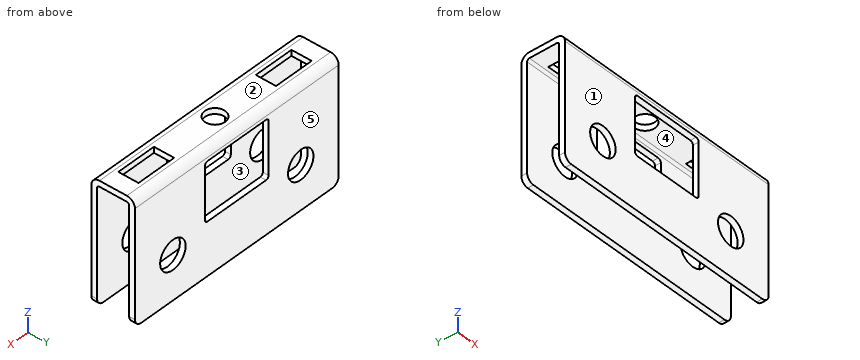
```python
from build123d import *

# Parameters (mm, degrees)
SKETCH1_W                      = 80
SKETCH1_H                      = 2
BASE_FLANGE1_DEPTH             = 5.55
EDGE_FLANGE1_STRIP_W           = 9.6
EDGE_FLANGE1_STRIP_H           = 2
EDGE_FLANGE1_STRIP_CUT_DEPTH   = 80
EDGE_FLANGE1_STRIP_2_W         = 9.6
EDGE_FLANGE1_STRIP_2_H         = 2
EDGE_FLANGE1_STRIP_CUT_2_DEPTH = 80
EDGE_FLANGE1_DEPTH             = 80
EDGE_FLANGE1_BEND_DEPTH        = 80
SKETCH12_R                     = 3.5
SKETCH12_W                     = 14
SKETCH12_H                     = 7
CUT_EXTRUDE1_DEPTH             = 59.561185951
SKETCH13_W                     = 25
SKETCH13_H                     = 20
CUT_EXTRUDE2_DEPTH             = 59.617574157
FILLET1_R                      = 1
FILLET2_R                      = 2.5
SKETCH15_R                     = 5
CUT_EXTRUDE3_DEPTH             = 59.617574157


# Sheet-metal steps are written as plain solids
with BuildPart() as part:
    # Sketch1 → Base-Flange1 (new, symmetric)
    with BuildSketch(Plane(origin=(0, 0, 0), x_dir=(1, 0, 0), z_dir=(0, 1, 0))):
        with Locations((0, -1)):
            Rectangle(SKETCH1_W, SKETCH1_H)
    extrude(amount=BASE_FLANGE1_DEPTH, both=True)

    # Edge-Flange1 strip (across the edge) → Edge-Flange1 strip cut (cut)
    with BuildSketch(Plane(origin=(40, -5.55, 0), x_dir=(0, 1, 0), z_dir=(-1, 0, 0))):
        with Locations((-4, -1)):
            Rectangle(EDGE_FLANGE1_STRIP_W, EDGE_FLANGE1_STRIP_H)
    extrude(amount=EDGE_FLANGE1_STRIP_CUT_DEPTH, mode=Mode.SUBTRACT)

    # Edge-Flange1 strip 2 (across the edge) → Edge-Flange1 strip cut 2 (cut)
    with BuildSketch(Plane(origin=(-40, 5.55, 0), x_dir=(0, -1, 0), z_dir=(1, 0, 0))):
        with Locations((-4, -1)):
            Rectangle(EDGE_FLANGE1_STRIP_2_W, EDGE_FLANGE1_STRIP_2_H)
    extrude(amount=EDGE_FLANGE1_STRIP_CUT_2_DEPTH, mode=Mode.SUBTRACT)

    # Edge-Flange1 section (across the edge) → Edge-Flange1 (add)
    with BuildSketch(Plane(origin=(40, -5.55, 0), x_dir=(0, 1, 0), z_dir=(-1, 0, 0))):
        with BuildLine():
            Line((-2, 0.8), (-2, 40.1))
            Line((-2, 40.1), (0, 40.1))
            Line((0, 40.1), (0, 0.8))
            ThreePointArc((0, 0.8), (0.234314575, 0.234314575), (0.8, 0))
            Line((0.8, 0), (0.8, -2))
            ThreePointArc((0.8, -2), (-1.179898987, -1.179898987), (-2, 0.8))
        make_face()
    extrude(amount=EDGE_FLANGE1_DEPTH)

    # Edge-Flange1 section 2 (across the edge) → Edge-Flange1 bend (add)
    with BuildSketch(Plane(origin=(-40, 5.55, 0), x_dir=(0, -1, 0), z_dir=(1, 0, 0))):
        with BuildLine():
            Line((-2, 0.8), (-2, 40.1))
            Line((-2, 40.1), (0, 40.1))
            Line((0, 40.1), (0, 0.8))
            ThreePointArc((0, 0.8), (0.234314575, 0.234314575), (0.8, 0))
            Line((0.8, 0), (0.8, -2))
            ThreePointArc((0.8, -2), (-1.179898987, -1.179898987), (-2, 0.8))
        make_face()
    extrude(amount=EDGE_FLANGE1_BEND_DEPTH)

    # Sketch12 → Cut-Extrude1 (cut, through all)
    with BuildSketch(Plane.XY.offset(2)):
        Circle(SKETCH12_R)
        with Locations((-27, 0)):
            Rectangle(SKETCH12_W, SKETCH12_H)
        with Locations((27, 0)):
            Rectangle(SKETCH12_W, SKETCH12_H)
    extrude(amount=-CUT_EXTRUDE1_DEPTH, mode=Mode.SUBTRACT)

    # Sketch13 → Cut-Extrude2 (cut, through all)
    with BuildSketch(Plane(origin=(0, 7.55, 0), x_dir=(1, 0, 0), z_dir=(0, 1, 0))):
        with Locations((0, 12)):
            Rectangle(SKETCH13_W, SKETCH13_H)
    extrude(amount=-CUT_EXTRUDE2_DEPTH, mode=Mode.SUBTRACT)

    # Fillet1
    fillet1_edges = [part.edges().sort_by_distance(p)[0] for p in [
        (-12.5, -6.55, -2),
        (-12.5, -6.55, -22),
        (12.5, -6.55, -22),
        (12.5, -6.55, -2),
        (-12.5, 6.55, -2),
        (-12.5, 6.55, -22),
        (12.5, 6.55, -22),
        (12.5, 6.55, -2),
    ]]
    fillet(fillet1_edges, radius=FILLET1_R)

    # Fillet2
    fillet2_edges = [part.edges().sort_by_distance(p)[0] for p in [
        (40, -6.55, -40.1),
        (-40, -6.55, -40.1),
        (-40, 6.55, -40.1),
        (40, 6.55, -40.1),
    ]]
    fillet(fillet2_edges, radius=FILLET2_R)

    # Sketch15 → Cut-Extrude3 (cut, through all)
    with BuildSketch(Plane.XZ.offset(7.55)):
        with Locations(Location((25.1, -25, 0), (0, 0, 270))):
            Circle(SKETCH15_R)
        with Locations(Location((-25.1, -25, 0), (0, 0, 270))):
            Circle(SKETCH15_R)
    extrude(amount=-CUT_EXTRUDE3_DEPTH, mode=Mode.SUBTRACT)


solid = part.part
```
Input: part model. Units: mm. Frame: model coordinates. Face numbers are marked on the shaded views. A direction names the side the tool comes from. Give positions to 0.01 mm unless a question says otherwise; leave off trailing zeros. Loops run counter-clockwise (first coordinate to the right, second up) from the corner with the lowest first, then second, coordinate; pieces in that order, holes last.
1) Section query A-A on z = -33. Return the cut outline in (x, y), and give its area (3 significant figures).
A:
outline: (-40, -7.55) - (40, -7.55) - (40, -5.55) - (-40, -5.55) - close; (-40, 5.55) - (40, 5.55) - (40, 7.55) - (-40, 7.55) - close
area: 320 mm2
2) Reachability of the marked faces 4 and 5 from +Z, -Z, +X, -X, +Y, -Y: full face, straight path, thin tool, end or side. Return the list, or none.
A:
face 4: -Z, +X, -X
face 5: +Z, -Z, +X, -X, +Y
3) Mould query, pull axis Y, two halves, no side actions, for the marked faces 1, 2 and 3. Classes: released by +Y, released by -Y, zero draft, split by the parting line, or undercut.
A:
face 1: released by -Y
face 2: zero draft
face 3: undercut
4) Section query B-B on x = -25.1. Return the cut outline in (y, z), and give its area (3 significant figures).
A:
outline: (-7.55, -40.1) - (-5.55, -40.1) - (-5.55, -30) - (-7.55, -30) - close; (-7.55, -20) - (-5.55, -20) - (-5.55, -0.8) arc R0.8 cw to (-4.75, 0) - (-3.5, 0) - (-3.5, 2) - (-4.75, 2) arc R2.8 ccw to (-7.55, -0.8) - close; (3.5, 0) - (4.75, 0) arc R0.8 cw to (5.55, -0.8) - (5.55, -20) - (7.55, -20) - (7.55, -0.8) arc R2.8 ccw to (4.75, 2) - (3.5, 2) - close; (5.55, -40.1) - (7.55, -40.1) - (7.55, -30) - (5.55, -30) - close
area: 134 mm2
5) Contact query for flat-ended pins moving along their axis: pin 1 (12 mm diameter, centred on x = 4, z = -18.5, fed in from +Y); pin 2 (2 mm diameter, centred on x = 24.5, z = 0.5, fed in from -Y); pin 3 (7.5 mm diameter, centred on x = 19, y = -0.5, fed in from -Z); pin 4 (0.6 mm diameter, centred on x = -24, z = 1, fed in from -Y). Output: stop coordinate, or through.
A:
pin 1: stops at y = 7.55
pin 2: stops at y = -7.53
pin 3: stops at z = 0
pin 4: stops at y = -7.11
6) Line query: L1, parallel to X at y = -6.6, z = -25; L2, parallel to Y at x = -16, z = -1.5; L3, parallel to Z at x = -8.5, y = -4.75. Output: solid intervals per line, ascending.
A:
L1: x = -40 to -30.1, -20.1 to 20.1, 30.1 to 40
L2: y = -7.55 to -5.55, 5.55 to 7.55
L3: z = 0 to 2
7) Section query C-C on y = 0. Return the cut outline in (x, z), and give its area (3 significant figures).
A:
outline: (-40, 0) - (-34, 0) - (-34, 2) - (-40, 2) - close; (-20, 0) - (-3.5, 0) - (-3.5, 2) - (-20, 2) - close; (3.5, 0) - (20, 0) - (20, 2) - (3.5, 2) - close; (34, 0) - (40, 0) - (40, 2) - (34, 2) - close
area: 90.0 mm2
8) Section query D-D on z = -13.5. Return the cut outline in (x, y).
A:
outline: (-40, -7.55) - (-12.5, -7.55) - (-12.5, -5.55) - (-40, -5.55) - close; (-40, 5.55) - (-12.5, 5.55) - (-12.5, 7.55) - (-40, 7.55) - close; (12.5, -7.55) - (40, -7.55) - (40, -5.55) - (12.5, -5.55) - close; (12.5, 5.55) - (40, 5.55) - (40, 7.55) - (12.5, 7.55) - close
